Here's the drawing with two shaded views (mm, measured from the low corner). I have some questions. A direction names the side the tool comes from. Give positions to 0.01 mm unless a question says otherwise; leave off trailing zeros. Loops run counter-clockwise (first coordinate to the right, second up) from the corner with the lowest first, then second, coordinate; pieces in that order, holes last. Notation, with made-up numbers: M 64,71.5 L 77,71.5 A20 ccw 77,90.5 Z; hole C 43,65.5 d8. An arc over 180 degrees is marked long. Answer in a Markdown table with one row per item. Add a question column.
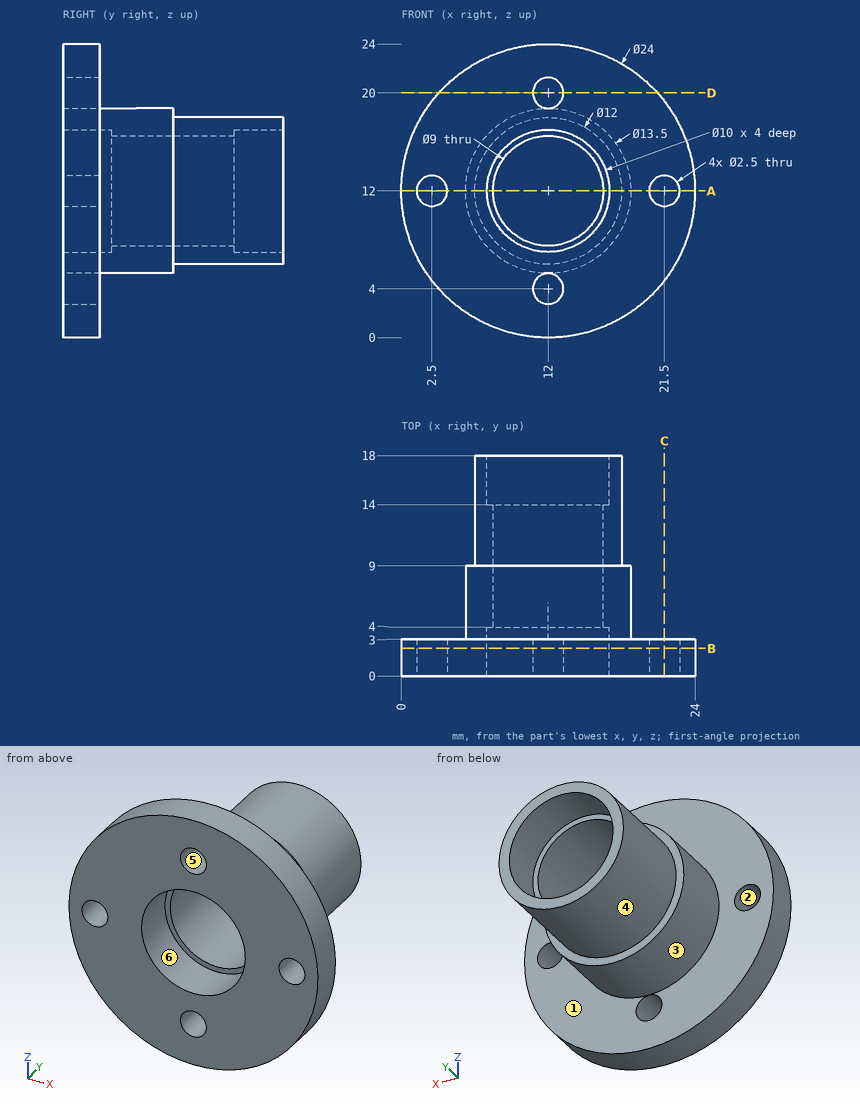
Item 1: Suppose I cut it at B-B (y = 2.25). List the corners of the cut face in (x, z) for me, then the cut area to 3 significant figures.
Item 2: Suppose I cut it at D-D (z = 20). List the corners of the cut face in (x, y) for me, then the cut area to 3 significant figures.
Item 3: Suppose I cut it at C-C (x = 21.5). List the corners of the cut face in (y, z) for me, then the cut area to 3 significant figures.
Item 4: I need wall thicknesses on L1, parallel to X at y = 1.1, z = 12; L2, parallel to X at y = 9.5, z = 12; L3, parallel to X at y = 16.5, z = 11.75. Which ranges of each line are inside material? Lowest first, please.
Item 5: If we mould it in two halves opening along Z, with no side actions, what happens to the marked faces 1, 2 and 3? For each: +Z half, -Z half, draft (parallel to the pull), parting line (faces both ways), or undercut.
Item 6: For the marked faces 4, 5 and 6, which set-ups out of +Z, -Z, +X, -X, +Y, -Y let a thin tool reach every point of the face, with its end or its side?
Item 7: Suppose I cut it at A-A (z = 12). Give the number of separate pieces and of enclosed holes in the cut face, then the cut area to 3 significant figures.
Item 8: For P1, Ø1.5, axis at x = 14.5, y = 2, coming from the -Z side; P2, Ø2, axis at x = 5.5, y = 6.5, coming from the +Z side; P3, Ø3, axis at x = 12, z = 20, coming from the +Y side, each with a flat end and sliding along its axis, tell me the tip position at first contact or that it passes through.
Values found:
| question | item | result |
|---|---|---|
| 1 | outline | C 12,12 d24; hole C 2.5,12 d2.5; hole C 12,12 d10; hole C 12,4 d2.5; hole C 12,20 d2.5; hole C 21.5,12 d2.5 |
| 1 | area | 354 mm² |
| 2 | outline | M 3.06,0 L 10.75,0 L 10.75,3 L 3.06,3 Z; M 13.25,0 L 20.94,0 L 20.94,3 L 13.25,3 Z |
| 2 | area | 46.2 mm² |
| 3 | outline | M 0,4.67 L 3,4.67 L 3,10.75 L 0,10.75 Z; M 0,13.25 L 3,13.25 L 3,19.33 L 0,19.33 Z |
| 3 | area | 36.5 mm² |
| 4 | L1 | 0 to 1.25, 3.75 to 7, 17 to 20.25, 22.75 to 24 |
| 4 | L2 | 6 to 7.5, 16.5 to 18 |
| 4 | L3 | 6.01 to 7.01, 16.99 to 17.99 |
| 5 | face 1 | draft |
| 5 | face 2 | undercut |
| 5 | face 3 | parting line |
| 6 | face 4 | +Y |
| 6 | face 5 | +Y, -Y |
| 6 | face 6 | -Y |
| 7 | separate pieces | 4 |
| 7 | enclosed holes | 0 |
| 7 | area | 76.0 mm² |
| 8 | P1 | z = 0.13 |
| 8 | P2 | z = 15.91 |
| 8 | P3 | y = 9 |
